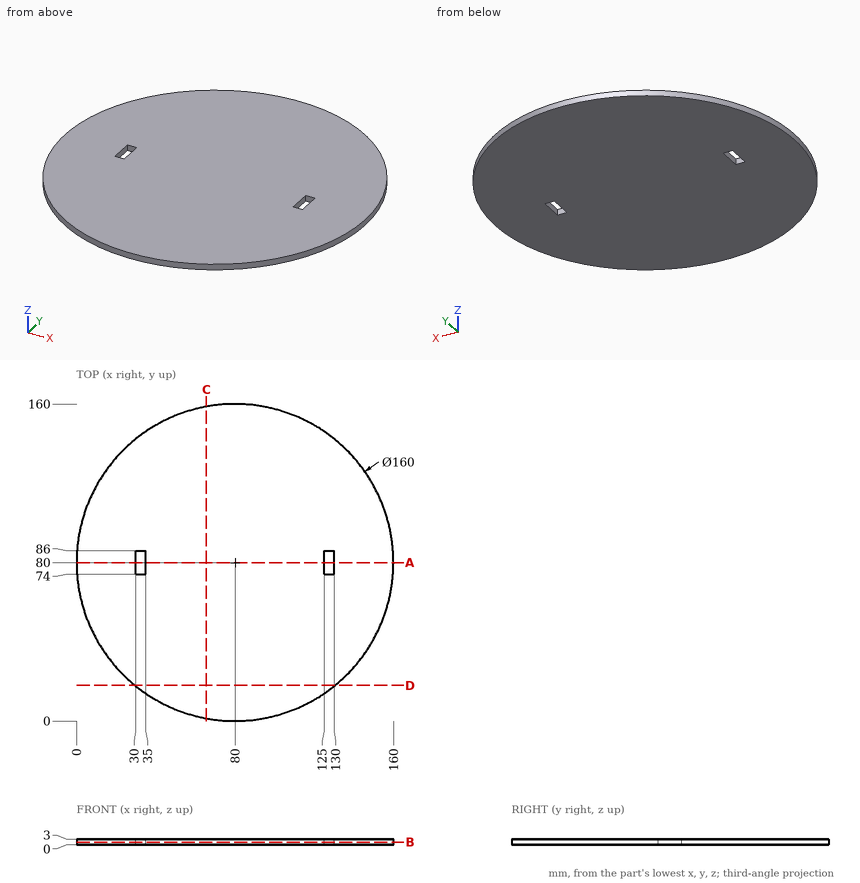
Job drawing, mm, ordinate dimensions from the low corner. One solid piece. Coordinates: 2 decimals unless noted, no trailing zeros. Order: outer loops, then holes, each group sorted by start corner. A loop starts at its lowest first (then second) coordinate and runs counter-clockwise, first axis right, second up. Notation, with made-up numbers: (52, -35) -> (73, -35) arc R18 cw to (73, -31) -> close; hole circle Ø6 at (21.25, 13). An arc over 180 degrees is marked (long way). Answer in a Markdown table with one row per item. Add a question column.
Q1. Band-saw the part on A-A, the plane y = 80. List the corners of the cut face in (x, z).
Q2. Drop flat-ended pins along their axis: pin 1 (1.5 mm diameter, centred on x = 126.5, z = 2, fed in from +Y); pin 2 (12 mm diameter, centred on x = 119.5, y = 47.5, fed in from -Z); pin 3 (1 mm diameter, centred on x = 132.5, z = 0.5, fed in from -Y); pin 4 (1 mm diameter, centred on y = 132.5, z = 2, fed in from +X). Give the stop position or say it passes through.
Q3. Band-saw the part on D-D, the plane y = 18. List the corners of the cut face in (x, z), then the cut area to 3 significant figures.
Q4. Band-saw the part on C-C, the plane x = 65.5. List the corners of the cut face in (y, z).
Q5. Wall check: line 1 along Y through (x, z) = (37, 2.2); line 2 along X through (y, z) = (43, 1.65); line 3 along Y through (x, z) = (75, 1.45). Give the ranges that are in metal, low to high. Write a range as [from, to].
Q6. Band-saw the part on B-B, the plane z = 1.45. List the corners of the cut face in (x, y).
Answers follow:
| question | item | result |
|---|---|---|
| 1 | outline | (0, 0) -> (30, 0) -> (30, 3) -> (0, 3) -> close; (35, 0) -> (125, 0) -> (125, 3) -> (35, 3) -> close; (130, 0) -> (160, 0) -> (160, 3) -> (130, 3) -> close |
| 2 | pin 1 | y = 145.63 |
| 2 | pin 2 | z = 0 |
| 2 | pin 3 | y = 19.21 |
| 2 | pin 4 | x = 140.79 |
| 3 | outline | (29.44, 0) -> (130.56, 0) -> (130.56, 3) -> (29.44, 3) -> close |
| 3 | area | 303 mm^2 |
| 4 | outline | (1.33, 0) -> (158.67, 0) -> (158.67, 3) -> (1.33, 3) -> close |
| 5 | line 1 | [12.54, 147.46] |
| 5 | line 2 | [9.07, 150.93] |
| 5 | line 3 | [0.16, 159.84] |
| 6 | outline | circle Ø160 at (80, 80); hole (30, 74) -> (35, 74) -> (35, 86) -> (30, 86) -> close; hole (125, 74) -> (130, 74) -> (130, 86) -> (125, 86) -> close |
